Here's how the part is built. I have some questions about the finished solid (model axes, mm). Face numbers are marked on the shaded views. A direction names the side the tool comes from. Coordinates: 2 decimals unless noted, no trailing zeros. Use a Markdown table: item, result. Add a question column.
Item 1: On a 3-axis mill with a long thin cutter (end or side, diameter ignored), from which of +Z, -Z, +X, -X, +Y, -Y can I reach the whole of each face in a straight line? I mean the marked faces 1 and 2. Say none if no direction works.
Item 2: If I drill on line 1 along Z through (x, y) = (0, -73); line 2 along Z through (x, y) = (10.16, 144); line 3 along Z through (x, y) = (0, -15), over which ranges is the centre line in solid material (lowest first)? Write a range as from..to.
Item 3: Imagine slicing it at A-A, the plane y = 163. Count the separate pieces of the cut face and the enclosed holes in it, and give its area (3 significant figures).
Item 4: Will these pins go through, and if not, where does the flat tip stop? pin 1 Ø21.5 at (x, z) = (-10.16, 17.6) entering from +Y; pin 2 Ø2 at (x, y) = (-61.5, -34) entering from +Z; pin 3 Ø18 at (x, z) = (12, -19) entering from +Y.
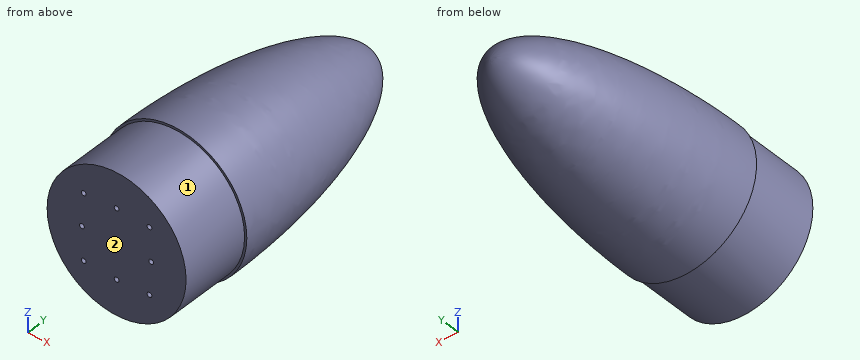
```python
from build123d import *

# Parameters (mm, degrees)
SKETCH2_R           = 75.9206
BOSS_EXTRUDE1_DEPTH = 76.2
SKETCH4_R           = 17.78
CUT_EXTRUDE1_DEPTH  = 96.52
CUT_EXTRUDE2_START  = 106.68
SKETCH5_R           = 8.255
CUT_EXTRUDE2_DEPTH  = 119.38
CUT_EXTRUDE3_START  = -25.4
SKETCH19_R          = 15.24
CUT_EXTRUDE3_DEPTH  = 101.6
SKETCH21_R          = 2.6035
CUT_EXTRUDE4_DEPTH  = 10.16
SKETCH22_R          = 2.6035
CUT_EXTRUDE5_DEPTH  = 10.16


with BuildPart() as part:
    # Sketch1 → Revolve1 (revolve)
    with BuildSketch(Plane.XY):
        with BuildLine():
            Line((78.359, 0), (0, 0))
            Line((0, 0), (0, 254))
            add(Edge.make_bspline(
                [(78.359, 0), (78.359, 0.547287489), (78.357845602, 1.649563618), (78.352650776, 3.586349875), (78.338796346, 5.988934596), (78.318010672, 8.352211569), (78.29028895, 10.745600888), (78.246958697, 13.731411826), (78.181061307, 17.311703382), (78.08386626, 21.490442467), (77.944822085, 26.264117007), (77.777683186, 31.037557631), (77.58229134, 35.809557456), (77.358460439, 40.580511863), (77.042853487, 46.542286246), (76.679080298, 52.501436144), (76.266448568, 58.457359127), (75.804102806, 64.409607399), (75.404015228, 69.168949637), (74.865626928, 75.114798701), (74.157385744, 82.243973993), (73.238266918, 90.551730955), (72.055740597, 100.030771811), (70.735528943, 109.491671534), (69.270929118, 118.931305028), (67.249996919, 130.699881306), (64.501732948, 144.763840427), (61.308555538, 158.735984092), (57.591049496, 172.577213574), (53.383025938, 186.275905479), (49.238746312, 198.044837449), (44.48323743, 209.587335711), (38.942884235, 220.71924179), (34.256173135, 228.693595393), (29.818710248, 235.095423042), (25.624249732, 240.182852143), (21.978892835, 243.926180276), (18.570150197, 246.859542723), (15.474349081, 249.076247661), (12.563405711, 250.785701438), (9.772327363, 252.083533871), (7.063069709, 253.028642362), (4.275373805, 253.686778481), (2.188006886, 253.939891173), (0.767171586, 253.999916555), (0, 254)],
                knots=[0.083290168, 0.083290168, 0.083290168, 0.083290168, 0.083290168, 0.091119674, 0.09894918, 0.106778686, 0.114608192, 0.122437698, 0.130267203, 0.145926215, 0.161585227, 0.177244239, 0.192903251, 0.208562263, 0.224221275, 0.239880287, 0.27119831, 0.286857322, 0.302516334, 0.318175346, 0.333834359, 0.365152383, 0.396470407, 0.42778843, 0.459106453, 0.490424474, 0.521742495, 0.584378539, 0.647014581, 0.678332609, 0.709650637, 0.772286631, 0.810589211, 0.841907031, 0.872607503, 0.893486158, 0.91262845, 0.928287274, 0.941044948, 0.952387223, 0.962498308, 0.97249612, 0.981348672, 0.989949856, 1, 1, 1, 1, 1], degree=4))
        make_face()
    revolve(axis=Axis((0, 254, 0), (0, -1, 0)))

    # Sketch2 → Boss-Extrude1 (add)
    with BuildSketch(Plane.XZ):
        Circle(SKETCH2_R)
    extrude(amount=BOSS_EXTRUDE1_DEPTH)

    # Sketch4 → Cut-Extrude1 (cut)
    with BuildSketch(Plane(origin=(0, 0, 0), x_dir=(1, 0, 0), z_dir=(0, 1, 0))):
        with Locations((48.26, 0)):
            Circle(SKETCH4_R)
        with Locations((0, -48.26)):
            Circle(SKETCH4_R)
        with Locations((-48.26, 0)):
            Circle(SKETCH4_R)
        with Locations((0, 48.26)):
            Circle(SKETCH4_R)
    extrude(amount=CUT_EXTRUDE1_DEPTH, mode=Mode.SUBTRACT)

    # Sketch5 → Cut-Extrude2 (cut)
    with BuildSketch(Plane(origin=(0, 0, 0), x_dir=(1, 0, 0), z_dir=(0, 1, 0)).offset(CUT_EXTRUDE2_START)):
        with Locations((20.32, 0)):
            Circle(SKETCH5_R)
        with Locations((10.16, -17.597636205)):
            Circle(SKETCH5_R)
        with Locations((-10.16, -17.597636205)):
            Circle(SKETCH5_R)
        with Locations((-20.32, 0)):
            Circle(SKETCH5_R)
        with Locations((-10.16, 17.597636205)):
            Circle(SKETCH5_R)
        with Locations((10.16, 17.597636205)):
            Circle(SKETCH5_R)
    extrude(amount=CUT_EXTRUDE2_DEPTH, mode=Mode.SUBTRACT)

    # Sketch6 → Cut-Revolve2 (revolve, cut)
    with BuildSketch(Plane.XY):
        Polygon((-30.48, 96.52), (-48.26, 117.709378876), (-48.26, 96.52), align=None)
    revolve(axis=Axis((-48.26, 96.52, 0), (0, -1, 0)), mode=Mode.SUBTRACT)

    # Sketch8 → Cut-Revolve4 (revolve, cut)
    with BuildSketch(Plane.XY.offset(48.26)):
        Polygon((0, 96.52), (17.78, 96.52), (0, 117.709378876), align=None)
    revolve(axis=Axis((0, 96.52, 48.26), (0, -1, 0)), mode=Mode.SUBTRACT)

    # Sketch9 → Cut-Revolve5 (revolve, cut)
    with BuildSketch(Plane.XY):
        Polygon((48.26, 96.52), (66.04, 96.52), (48.26, 117.709378876), align=None)
    revolve(axis=Axis((48.26, 96.52, 0), (0, -1, 0)), mode=Mode.SUBTRACT)

    # Sketch11 → Cut-Revolve6 (revolve, cut)
    with BuildSketch(Plane.XY.offset(-48.26)):
        Polygon((0, 96.52), (17.78, 96.52), (0, 117.709378876), align=None)
    revolve(axis=Axis((0, 96.52, -48.26), (0, -1, 0)), mode=Mode.SUBTRACT)

    # Sketch12 → Cut-Revolve7 (revolve, cut)
    with BuildSketch(Plane.XY):
        Polygon((-20.32, 226.06), (-12.065, 226.06), (-20.32, 235.897925907), align=None)
    revolve(axis=Axis((-20.32, 226.06, 0), (0, -1, 0)), mode=Mode.SUBTRACT)

    # Sketch14 → Cut-Revolve8 (revolve, cut)
    with BuildSketch(Plane.XY):
        Polygon((20.32, 226.06), (28.575, 226.06), (20.32, 235.897925907), align=None)
    revolve(axis=Axis((20.32, 235.897925907, 0), (0, -1, 0)), mode=Mode.SUBTRACT)

    # Sketch15 → Cut-Revolve9 (revolve, cut)
    with BuildSketch(Plane.XY.offset(17.597636205)):
        Polygon((-10.16, 226.06), (-1.905, 226.06), (-10.16, 235.897925907), align=None)
    revolve(axis=Axis((-10.16, 226.06, 17.597636205), (0, -1, 0)), mode=Mode.SUBTRACT)

    # Sketch16 → Cut-Revolve10 (revolve, cut)
    with BuildSketch(Plane.XY.offset(17.597636205)):
        Polygon((10.16, 226.06), (18.415, 226.06), (10.16, 235.897925907), align=None)
    revolve(axis=Axis((10.16, 235.897925907, 17.597636205), (0, -1, 0)), mode=Mode.SUBTRACT)

    # Sketch17 → Cut-Revolve11 (revolve, cut)
    with BuildSketch(Plane.XY.offset(-17.597636205)):
        Polygon((10.16, 226.06), (18.415, 226.06), (10.16, 235.897925907), align=None)
    revolve(axis=Axis((10.16, 235.897925907, -17.597636205), (0, -1, 0)), mode=Mode.SUBTRACT)

    # Sketch18 → Cut-Revolve12 (revolve, cut)
    with BuildSketch(Plane.XY.offset(-17.597636205)):
        Polygon((-10.16, 226.06), (-1.905, 226.06), (-10.16, 235.897925907), align=None)
    revolve(axis=Axis((-10.16, 235.897925907, -17.597636205), (0, -1, 0)), mode=Mode.SUBTRACT)

    # Sketch19 → Cut-Extrude3 (cut)
    with BuildSketch(Plane(origin=(0, 0, 0), x_dir=(1, 0, 0), z_dir=(0, 1, 0)).offset(CUT_EXTRUDE3_START)):
        Circle(SKETCH19_R)
    extrude(amount=CUT_EXTRUDE3_DEPTH, mode=Mode.SUBTRACT)

    # Sketch20 → Cut-Revolve13 (revolve, cut)
    with BuildSketch(Plane.XY):
        Polygon((0, 76.2), (15.24, 76.2), (0, 94.362324751), align=None)
    revolve(axis=Axis((0, 270.51, 0), (0, -1, 0)), mode=Mode.SUBTRACT)

    # Sketch21 → Cut-Extrude4 (cut)
    with BuildSketch(Plane.XZ.offset(76.2)):
        with Locations((-37.81298, 0)):
            Circle(SKETCH21_R)
        with Locations((0, 37.81298)):
            Circle(SKETCH21_R)
        with Locations((37.81298, 0)):
            Circle(SKETCH21_R)
        with Locations((0, -37.81298)):
            Circle(SKETCH21_R)
    extrude(amount=-CUT_EXTRUDE4_DEPTH, mode=Mode.SUBTRACT)

    # Sketch22 → Cut-Extrude5 (cut)
    with BuildSketch(Plane.XZ.offset(76.2)):
        with Locations((-35.921024484, -35.921024484)):
            Circle(SKETCH22_R)
        with Locations((-35.921024484, 35.921024484)):
            Circle(SKETCH22_R)
        with Locations((35.921024484, 35.921024484)):
            Circle(SKETCH22_R)
        with Locations((35.921024484, -35.921024484)):
            Circle(SKETCH22_R)
    extrude(amount=-CUT_EXTRUDE5_DEPTH, mode=Mode.SUBTRACT)

    # Sketch3 → Cut-Revolve1 (revolve, cut)
    with BuildSketch(Plane.XY):
        with BuildLine():
            Line((0, 0), (50.695639171, 0))
            ThreePointArc((50.695639171, 0), (37.521185782, 66.292890616), (0, 122.510985441))
            Line((0, 122.510985441), (0, 0))
        make_face()
    revolve(axis=Axis((0, 270.51, 0), (0, -1, 0)), mode=Mode.SUBTRACT)


solid = part.part
```
Ans:
| question | item | result |
|---|---|---|
| 1 | face 1 | -Y |
| 1 | face 2 | +Z, -Z, +X, -X, -Y |
| 2 | line 1 | z = -75.92..-40.42, -35.21..35.21, 40.42..75.92 |
| 2 | line 2 | z = -63.74..-25.85, -9.34..9.34, 25.85..63.74 |
| 2 | line 3 | z = -75.92..-15.24, 15.24..75.92 |
| 3 | separate pieces | 1 |
| 3 | enclosed holes | 6 |
| 3 | area | 10,100 mm^2 |
| 4 | pin 1 | stops at y = 252.1 |
| 4 | pin 2 | stops at z = 45.87 |
| 4 | pin 3 | stops at y = 250.22 |
